The model under review builds one solid part; all positions refer to its coordinate system, in mm. Face numbers are marked on the shaded views. A direction names the side the tool comes from. Coordinates: 2 decimals unless noted, no trailing zeros. Loops run counter-clockwise (first coordinate to the right, second up) from the corner with the lowest first, then second, coordinate; pieces in that order, holes last. Notation, with made-up numbers: (88, 7.5) - (143, 7.5) arc R15 ccw to (143, 31.5) - close; hole circle Ø5 at (87.25, 9.25). An arc over 180 degrees is marked (long way). Answer in a Markdown table with one row per item. Add a question column.
(1) Machinability: for the marked faces 1 and 2, which of the approach directions +Z, -Z, +X, -X, +Y, -Y give a long, thin tool a straight path to every point of the face, cutting with its end or side? Answer none if there is none.
(2) For line 1 along Y through (x, z) = (-3, 0); line 2 along Z through (x, y) = (-11.25, -0.25); line 3 along X through (y, z) = (2, -6.75), list the stretches that pass through material, from the lowest coordinate up.
(3) We need section C-C on x = -11. Write out the cut boundary in (y, z).
(4) For P1, Ø10, axis at x = -1.5, y = 4.5, coming from the -Z side; P2, Ø8.5, axis at y = 0, z = 0, coming from the -X side; P3, Ø3, axis at x = 3, z = -6.5, coming from the -Y side, all flat-tipped, find the tip position at first contact; note any pin that passes through.
(5) We need section A-A on x = -1.5. Write out the cut boundary in (y, z), plus the area to 3 significant figures.
(6) Mouldability with a two-part tool opening along Y and no side actions: class the marked faces 3, 4, 5 and 6 as +Y half, -Y half, draft (parallel to the pull), parting line (faces both ways), or undercut.
from build123d import *
from build123d.topology import SkipClean

# Parameters (mm, degrees)
CUT_SWEEP1_PITCH = 1.411111111


with BuildPart() as part:
    # Sketch1 → Revolve1 (revolve)
    with BuildSketch(Plane.XY, mode=Mode.PRIVATE) as revolve1_sk:
        Polygon((-13.0937, 8.6614), (-13.0937, 7.4803), (-8.172486984, 3.7719), (13.0937, 3.7719), (13.0937, 4.337685), (13.0937, 7.14375), (9.369925973, 7.14375), (-1.0287, 7.14375), (-1.0287, 7.1374), (-7.5311, 7.1374), (-7.5311, 8.6614), align=None)
    revolve(revolve1_sk.sketch.rotate(Axis((-13.0937, 0, 0), (1, 0, 0)), 90), axis=Axis((-13.0937, 0, 0), (1, 0, 0)))

    # Cut-Sweep1: the profile of Sketch4 profile screwed along a right-hand helix of 10.008 turns, 8 arcs to a turn; built about Z, then put on its axis
    cut_sweep1_z = Axis((0, 0, 0), (0, 0, 1))
    cut_sweep1_corners = [(7.14435, 0, 0.00034641), (7.14435, 0, -1.235068632), (6.227206448, 0, -0.705555556), (6.227206448, 0, -0.529166667)]
    with BuildLine(mode=Mode.PRIVATE) as cut_sweep1_profile:
        Line(cut_sweep1_corners[0], cut_sweep1_corners[1])
        Line(cut_sweep1_corners[1], cut_sweep1_corners[2])
        Line(cut_sweep1_corners[2], cut_sweep1_corners[3])
        Line(cut_sweep1_corners[3], cut_sweep1_corners[0])
    cut_sweep1_cap = Face(cut_sweep1_profile.wire())
    cut_sweep1_turn_angles = [0, 22.5, 45, 67.5, 90, 112.5, 135, 157.5, 180, 202.5, 225, 247.5, 270, 292.5, 315, 337.5, 360]
    cut_sweep1_turn_weights = [1, 0.9238795325112867, 1, 0.9238795325112867, 1, 0.9238795325112867, 1, 0.9238795325112867, 1, 0.9238795325112867, 1, 0.9238795325112867, 1, 0.9238795325112867, 1, 0.9238795325112867, 1]
    cut_sweep1_turn_rails = [Edge.make_bspline([Vector(p[0], p[1], 0).rotate(cut_sweep1_z, cut_sweep1_turn_angles[k]) / cut_sweep1_turn_weights[k] + Vector(0, 0, p[2] + CUT_SWEEP1_PITCH * cut_sweep1_turn_angles[k] / 360) for k in range(17)], [0, 0, 0, 1, 1, 2, 2, 3, 3, 4, 4, 5, 5, 6, 6, 7, 7, 8, 8, 8], 2, cut_sweep1_turn_weights) for p in cut_sweep1_corners]
    cut_sweep1_turn_sides = [Face.make_surface_from_curves(cut_sweep1_turn_rails[p[0]], cut_sweep1_turn_rails[p[1]]) for p in [(0, 1), (1, 2), (2, 3), (3, 0)]]
    cut_sweep1_last_angles = [3600, 3601.44, 3602.88]
    cut_sweep1_last_weights = [1, 0.9996841892832969, 1]
    cut_sweep1_last_rails = [Edge.make_bspline([Vector(p[0], p[1], 0).rotate(cut_sweep1_z, cut_sweep1_last_angles[k]) / cut_sweep1_last_weights[k] + Vector(0, 0, p[2] + CUT_SWEEP1_PITCH * cut_sweep1_last_angles[k] / 360) for k in range(3)], [0, 0, 0, 1, 1, 1], 2, cut_sweep1_last_weights) for p in cut_sweep1_corners]
    cut_sweep1_last_sides = [Face.make_surface_from_curves(cut_sweep1_last_rails[p[0]], cut_sweep1_last_rails[p[1]]) for p in [(0, 1), (1, 2), (2, 3), (3, 0)]]
    cut_sweep1 = Plane(origin=(13.0937, 0, 0), x_dir=(0, 1, 0), z_dir=(-1, 0, 0)) * Solid(Shell([*[p.moved(Location((0, 0, CUT_SWEEP1_PITCH * i))) for i in range(10) for p in cut_sweep1_turn_sides], *cut_sweep1_last_sides, cut_sweep1_cap, cut_sweep1_cap.rotate(cut_sweep1_z, 3602.88).moved(Location((0, 0, CUT_SWEEP1_PITCH * 3602.88 / 360)))]))
    add(cut_sweep1, mode=Mode.SUBTRACT)

    # Sketch5 → Cut-Revolve1 (revolve, cut)
    with BuildSketch(Plane.XY, mode=Mode.PRIVATE) as cut_revolve1_sk:
        Polygon((13.0937, 4.337685), (10.653634224, 6.176406448), (9.242523113, 6.176406448), (8.275179561, 7.14375), (13.0937, 7.14375), align=None)
        Polygon((-1.0287, 7.14375), (-1.0287, 6.176406448), (0.382411111, 6.176406448), (1.349754663, 7.14375), align=None)
    revolve(cut_revolve1_sk.sketch.rotate(Axis((0, 0, 0), (-1, 0, 0)), 90), axis=Axis((0, 0, 0), (-1, 0, 0)), mode=Mode.SUBTRACT)

    # Sketch6 → Revolve2 (revolve)
    with SkipClean():  # the faces are left unmerged after this step: merging them gives an invalid solid
        with BuildSketch(Plane.XY, mode=Mode.PRIVATE) as revolve2_sk:
            Polygon((1.349754663, 7.14375), (0.382411111, 6.176406448), (9.242523113, 6.176406448), (8.275179561, 7.14375), align=None)
        revolve(revolve2_sk.sketch.rotate(Axis((0, 0, 0), (-1, 0, 0)), 90), axis=Axis((0, 0, 0), (-1, 0, 0)))
    add(part.part.scale(1), mode=Mode.REPLACE)  # the faces are merged on a copy


solid = part.part
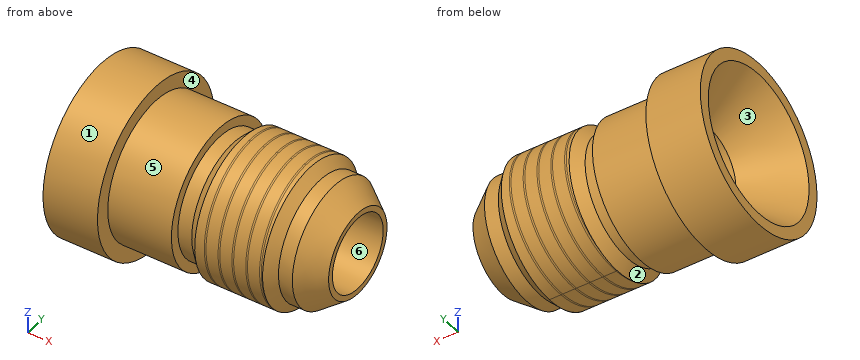
Outcome:
| question | item | result |
|---|---|---|
| 1 | face 1 | +X, -X |
| 1 | face 2 | none |
| 2 | line 1 | -7.14 to -3.77, 3.77 to 7.14 |
| 2 | line 2 | -8.66 to -6.09, 6.09 to 8.66 |
| 2 | line 3 | -12.51 to -1.03, 1.25 to 8.38 |
| 3 | outline | circle Ø17.32 at (0, 0); hole circle Ø11.81 at (0, 0) |
| 4 | P1 | z = -7.14 |
| 4 | P2 | x = -8.81 |
| 4 | P3 | y = -5.1 |
| 5 | outline | circle Ø14.27 at (0, 0); hole circle Ø7.54 at (0, 0) |
| 5 | area | 115 mm² |
| 6 | face 3 | undercut |
| 6 | face 4 | draft |
| 6 | face 5 | parting line |
| 6 | face 6 | undercut |
